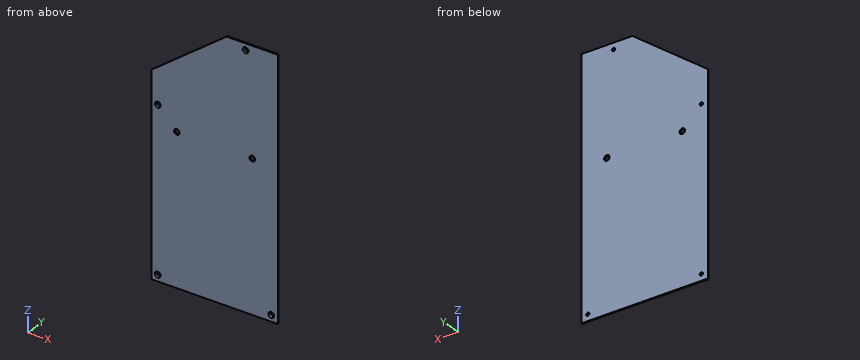
```python
from build123d import *

# Parameters (mm, degrees)
F1_DEPTH       = 2
F2_D           = 8.5
F2_DEPTH       = 15.75
F2_TIP         = 2.5536576309
F3_D           = 4.4
F3_CSINK_D     = 8.96
F3_CSINK_ANGLE = 90


with BuildPart() as f1:
    # F0 (on Front) → F1 (new body)
    with BuildSketch(Plane.XZ):
        Polygon((-180.7669961075, 124.533562243), (-180.7669961075, -183.466437757), (15.2330038925, -183.466437757), (15.2330038925, 212.533562243), (-63.9870518049, 212.533562243), align=None)
    extrude(amount=-F1_DEPTH)

    # F2
    with Locations(Plane.XZ):
        with Locations((-141.2669961075, 46.533562243), (-24.2669961075, 46.533562243)):
            Hole(F2_D / 2, depth=F2_DEPTH)
            with Locations((0, 0, -(F2_DEPTH + F2_TIP / 2))):  # 118° drill point
                Cone(0, F2_D / 2, F2_TIP, mode=Mode.SUBTRACT)

    # F3 (through all)
    with Locations(Plane.XZ):
        with Locations((-170.7669961075, 76.533562243), (-34.7669961075, 202.533562243), (5.2330038925, -173.466437757), (-170.7669961075, -173.466437757)):
            CounterSinkHole(F3_D / 2, F3_CSINK_D / 2, counter_sink_angle=F3_CSINK_ANGLE)


solid = f1.part
```
Design review of the part built by this model. Coordinates are the model's own, in mm. Round coordinates to 2 decimals unless told otherwise and drop trailing zeros. Order: outer loops, then holes, each group sorted by start corner. A loop starts at its lowest first (then second) coordinate and runs counter-clockwise, first axis right, second up. Notation, with made-up numbers: M 13,-7.75 L 46,-7.75 A19 ccw 46,-2.75 Z; hole C 9.25,22.5 d2. An arc over 180 degrees is marked long. Put each result on its own line as item: value.
Q1. Consider section A-A (y = 0.65). State the section outline as (x, z) points.
Reported:
outline: M -180.77,-183.47 L 15.23,-183.47 L 15.23,212.53 L -63.99,212.53 L -180.77,124.53 Z; hole C -170.77,-173.47 d7.66; hole C -170.77,76.53 d7.66; hole C -141.27,46.53 d8.5; hole C -34.77,202.53 d7.66; hole C -24.27,46.53 d8.5; hole C 5.23,-173.47 d7.66
Q2. Consider section C-C (x = -122.5). State the section outline as (y, z) points.
Reported:
outline: M 0,-183.47 L 2,-183.47 L 2,168.44 L 0,168.44 Z
Q3. Consider section B-B (z = 137.5). State the section outline as (x, y) points.
Reported:
outline: M -163.56,0 L 15.23,0 L 15.23,2 L -163.56,2 Z
Q4. To check wall thickness, follow line 1 (X direction, y = 1.7, z = 46); line 2 (Z direction, x = -64, y = 1.35); line 3 (Z direction, x = -138, y = 1.35). State the ranges of each line that lie inside material, in increasing order.
Reported:
line 1: -180.77 to -145.48, -137.05 to -28.48, -20.05 to 15.23
line 2: -183.47 to 212.52
line 3: -183.47 to 43.82, 49.25 to 156.76
